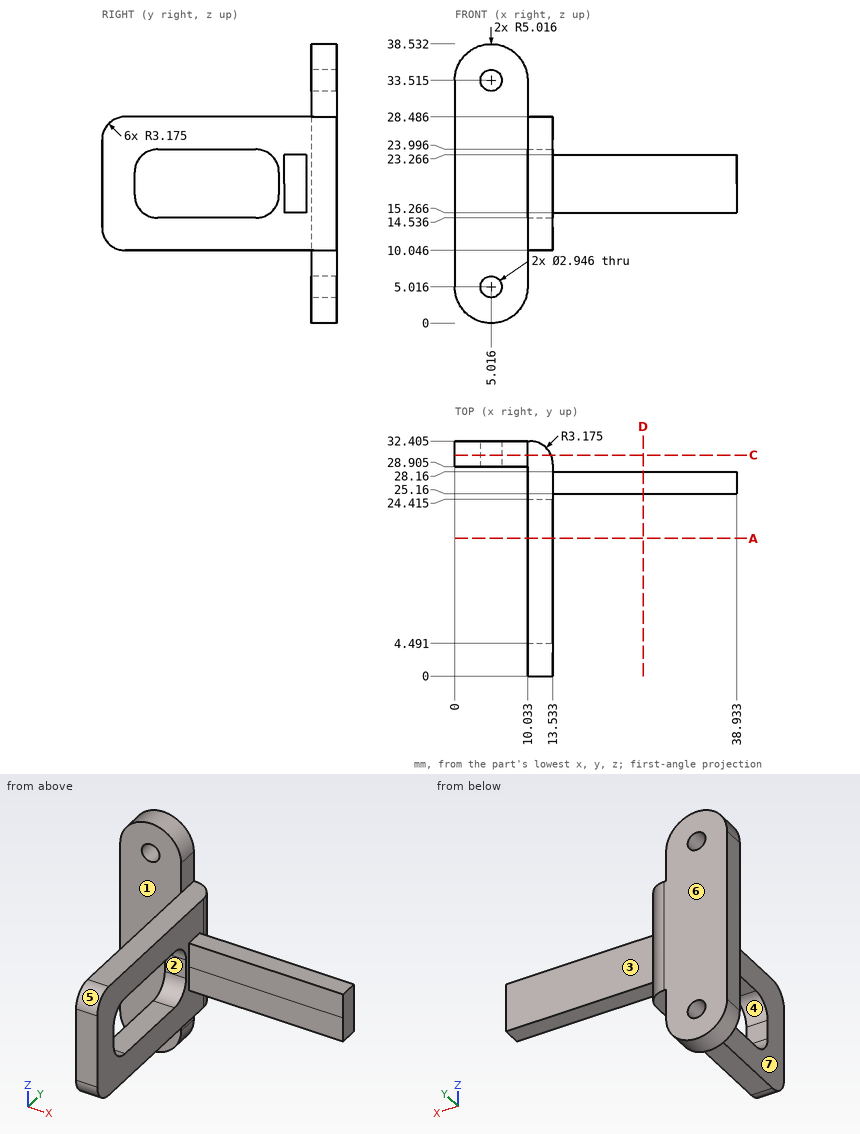
Input: dimensioned drawing with shaded views. Units: mm. Origin: part minimum x, y, z. A direction names the side the tool comes from. Round coordinates to 2 decimals unless told otherwise and drop trailing zeros. Order: outer loops, then holes, each group sorted by start corner. A loop starts at its lowest first (then second) coordinate and runs counter-clockwise, first axis right, second up.
Q1. Section C-C, the plane y = 30.5. Output: boundary loops of the cut face in (x, z) (1 decimal), and give its area (3 significant figures).
Result sheet:
outline: (0, 5) arc R5 ccw to (10, 5) - (10, 10) - (13.3, 10) - (13.3, 28.5) - (10, 28.5) - (10, 33.5) arc R5 ccw to (0, 33.5) - close; hole circle Ø2.9 at (5, 5); hole circle Ø2.9 at (5, 33.5)
area: 411 mm2
Q2. Section D-D, the plane x = 26. Output: boundary loops of the cut face in (y, z).
Result sheet:
outline: (25.16, 15.27) - (28.16, 15.27) - (28.16, 23.27) - (25.16, 23.27) - (25.16, 19.27) - close
Q3. Mould query, pull axis Y, two halves, no side actions, for the marked faces 4, 5, 6 and 7. Classes: released by +Y, released by -Y, zero draft, split by the parting line, or undercut.
Result sheet:
face 4: undercut
face 5: released by -Y
face 6: released by +Y
face 7: zero draft
Q4. Section A-A, the plane y = 19. Output: boundary loops of the cut face in (x, z) (1 decimal).
Result sheet:
outline: (10, 10) - (13.5, 10) - (13.5, 14.5) - (10, 14.5) - close; (10, 24) - (13.5, 24) - (13.5, 28.5) - (10, 28.5) - close
Q5. Pin query (flat end, axial travel): pin 1 (6 mm diameter, centred on x = 5.5, z = 28, fed in from -Y) (1 decimal); pin 2 (3 mm diameter, centred on x = 11, y = 15, fed in from -Z); pin 3 (12 mm diameter, centred on y = 21.5, z = 18, fed in from -X); pin 4 (8 mm diameter, centred on x = 7, z = 16.5, fed in from -Y). Return the tip coordinate at first contact, or that it passes through.
Result sheet:
pin 1: stops at y = 28.9
pin 2: stops at z = 10.05
pin 3: stops at x = 10.03
pin 4: stops at y = 0
Q6. Material intervals for probe 1 along Y at (x, z) = (33, 20); probe 2 along X at (y, z) = (30.5, 4.5) (1 decimal); probe 3 along X at (y, z) = (24.5, 17.5), sorted ascending.
Result sheet:
probe 1: y = 25.16 to 28.16
probe 2: x = 0 to 3.6, 6.4 to 10
probe 3: x = 10.03 to 13.53
Q7. Access query for the marked faces 1, 2 and 3. Directions: +Z, -Z, +X, -X, +Y, -Y. A direction counts if a zero-diameter tool reaches every point of the face in a straight line with its end or side. Return the directions, or none.
Result sheet:
face 1: +Z, -Z, -X, -Y
face 2: +X, -X
face 3: +Z, -Z, +X, +Y
